Model file for the job. Use its own axes, mm. Coordinates: 2 decimals unless noted, no trailing zeros. Order: outer loops, then holes, each group sorted by start corner. A loop starts at its lowest first (then second) coordinate and runs counter-clockwise, first axis right, second up. Notation, with made-up numbers: M -28,83.5 L 1,83.5 A17 ccw 1,108.5 Z; hole C -9.5,13 d6. An arc over 180 degrees is marked long. Return JSON: item names as keys, results as strings.
Autodesk Inventor part; units mm, degrees
ref_plane "Zplus_face" through (0, 0, 1.5875) normal (0, 0, 1) x (1, 0, 0)
ref_plane "Work Plane_ConnX" through (-32, 0, 0) normal (1, 0, 0) x (0, 1, 0)
ref_plane "Work Plane_ConnY" through (0, 0, 0) normal (0, 1, 0) x (-1, 0, 0)
sketch "AL_spacer_contact_Zminus" plane through (0, 0, 0) normal (0, 0, 1) x (1, 0, 0)
  circle A0 centre (39.5, 39.5) radius 3.175
  circle A1 centre (39.5, -39.5) radius 3.175
  circle A2 centre (-39.5, -39.5) radius 3.175
  circle A3 centre (-39.5, 39.5) radius 3.175
  point P0 (0, 0)
  dimension "d145" = 0
  dimension "d228" = 39.5
  dimension "d229" = 39.5
  dimension "d230" = 39.5
  dimension "d231" = 39.5
  dimension "d232" = 39.5
  dimension "d233" = 39.5
  dimension "d234" = 39.5
  dimension "d235" = 39.5
  dimension "d236" = 6.35
sketch "Delrin_stayout_Zminus" plane through (0, 0, 0) normal (0, 0, 1) x (1, 0, 0)
  line L0 (47.5, 39.5) -> (47.5, 31)
  line L1 (47.5, 31) -> (39.5, 31)
  line L2 (39.5, 31) -> (31, 39.5)
  line L3 (31, 39.5) -> (31, 47.5)
  line L4 (31, 47.5) -> (39.5, 47.5)
  line L5 (39.5, 47.5) -> (47.5, 39.5)
  line L6 (-39.5, 47.5) -> (-47.5, 39.5)
  line L7 (-47.5, 39.5) -> (-47.5, 31)
  line L8 (-47.5, 31) -> (-39.5, 31)
  line L9 (-39.5, 31) -> (-31, 39.5)
  line L10 (-31, 39.5) -> (-31, 47.5)
  line L11 (-31, 47.5) -> (-39.5, 47.5)
  line L12 (47.5, -39.5) -> (39.5, -47.5)
  line L13 (39.5, -47.5) -> (31, -47.5)
  line L14 (31, -47.5) -> (31, -39.5)
  line L15 (31, -39.5) -> (39.5, -31)
  line L16 (39.5, -31) -> (47.5, -31)
  line L17 (47.5, -31) -> (47.5, -39.5)
  line L18 (-39.5, -47.5) -> (-47.5, -39.5)
  line L19 (-47.5, -39.5) -> (-47.5, -31)
  line L20 (-47.5, -31) -> (-39.5, -31)
  line L21 (-39.5, -31) -> (-31, -39.5)
  line L22 (-31, -39.5) -> (-31, -47.5)
  line L23 (-31, -47.5) -> (-39.5, -47.5)
  point P0 (0, 0)
  dimension "d243" = 16.5
  dimension "d244" = 8
  dimension "d245" = 8.5
  dimension "d246" = 16.5
  dimension "d247" = 47.5
  dimension "d248" = 47.5
  dimension "d249" = 47.5
  dimension "d250" = 47.5
  dimension "d251" = 47.5
  dimension "d252" = 47.5
  dimension "d253" = 47.5
  dimension "d254" = 47.5
sketch "Nub_stayout_Zminus" plane through (0, 0, 0) normal (0, 0, 1) x (1, 0, 0)
  line L0 (29, 47.5) -> (39.5, 47.5)
  line L1 (39.5, 47.5) -> (47.5, 39.5)
  line L2 (47.5, 39.5) -> (47.5, 29)
  line L3 (47.5, 29) -> (42, 29)
  line L4 (42, 29) -> (42, 40.4125)
  line L5 (40.4125, 42) -> (29, 42)
  line L6 (29, 42) -> (29, 47.5)
  arc A0 (42, 40.4125) -> (40.4125, 42) centre (40.4125, 40.4125) ccw
  line L7 (-29, 47.5) -> (-39.5, 47.5)
  line L8 (-39.5, 47.5) -> (-47.5, 39.5)
  line L9 (-47.5, 39.5) -> (-47.5, 29)
  line L10 (-47.5, 29) -> (-42, 29)
  line L11 (-42, 29) -> (-42, 40.4125)
  line L12 (-40.4125, 42) -> (-29, 42)
  line L13 (-29, 42) -> (-29, 47.5)
  arc A1 (-40.4125, 42) -> (-42, 40.4125) centre (-40.4125, 40.4125) ccw
  line L14 (-47.5, -29) -> (-42, -29)
  line L15 (-42, -29) -> (-42, -40.4125)
  line L16 (-40.4125, -42) -> (-29, -42)
  line L17 (-29, -42) -> (-29, -47.5)
  line L18 (-29, -47.5) -> (-39.5, -47.5)
  line L19 (-39.5, -47.5) -> (-47.5, -39.5)
  line L20 (-47.5, -39.5) -> (-47.5, -29)
  arc A2 (-42, -40.4125) -> (-40.4125, -42) centre (-40.4125, -40.4125) ccw
  line L21 (47.5, -29) -> (42, -29)
  line L22 (42, -29) -> (42, -40.4125)
  line L23 (40.4125, -42) -> (29, -42)
  line L24 (29, -42) -> (29, -47.5)
  line L25 (29, -47.5) -> (39.5, -47.5)
  line L26 (39.5, -47.5) -> (47.5, -39.5)
  line L27 (47.5, -39.5) -> (47.5, -29)
  arc A3 (40.4125, -42) -> (42, -40.4125) centre (40.4125, -40.4125) ccw
  point P0 (0, 0)
  dimension "d255" = 1.5875
  dimension "d256" = 18.5
  dimension "d257" = 8
  dimension "d258" = 5.5
  dimension "d259" = 47.5
  dimension "d260" = 47.5
  dimension "d264" = 1.5875
  dimension "d265" = 47.5
  dimension "d266" = 47.5
  dimension "d267" = 1.5875
  dimension "d268" = 47.5
  dimension "d269" = 47.5
  dimension "d270" = 1.5875
  dimension "d271" = 47.5
  dimension "d272" = 47.5
ref_plane "Zplus_face" through (0, 0, 1.5875) normal (0, 0, 1) x (1, 0, 0)
sketch "AL_spacer_contact_Zplus" plane through (0, 0, 1.5875) normal (0, 0, 1) x (1, 0, 0)
  circle A0 centre (-39.5, 39.5) radius 3.175
  circle A1 centre (-39.5, -39.5) radius 3.175
  circle A2 centre (39.5, -39.5) radius 3.175
  circle A3 centre (39.5, 39.5) radius 3.175
  point P0 (0, 0)
  dimension "d129" = 39.5
  dimension "d130" = 39.5
  dimension "d131" = 39.5
  dimension "d132" = 39.5
  dimension "d133" = 6.35
sketch "Delrin_stayout_Zplus" plane through (0, 0, 1.5875) normal (0, 0, 1) x (1, 0, 0)
  line L0 (47.5, -31) -> (47.5, -39.5)
  line L1 (47.5, -39.5) -> (39.5, -47.5)
  line L2 (39.5, -47.5) -> (31, -47.5)
  line L3 (31, -47.5) -> (31, -39.5)
  line L4 (31, -39.5) -> (39.5, -31)
  line L5 (39.5, -31) -> (47.5, -31)
  line L6 (47.5, 31) -> (47.5, 39.5)
  line L7 (47.5, 39.5) -> (39.5, 47.5)
  line L8 (39.5, 47.5) -> (31, 47.5)
  line L9 (31, 47.5) -> (31, 39.5)
  line L10 (31, 39.5) -> (39.5, 31)
  line L11 (39.5, 31) -> (47.5, 31)
  line L12 (-39.5, 47.5) -> (-47.5, 39.5)
  line L13 (-47.5, 39.5) -> (-47.5, 31)
  line L14 (-47.5, 31) -> (-39.5, 31)
  line L15 (-39.5, 31) -> (-31, 39.5)
  line L16 (-31, 39.5) -> (-31, 47.5)
  line L17 (-31, 47.5) -> (-39.5, 47.5)
  line L18 (-47.5, -39.5) -> (-39.5, -47.5)
  line L19 (-39.5, -47.5) -> (-31, -47.5)
  line L20 (-31, -47.5) -> (-31, -39.5)
  line L21 (-31, -39.5) -> (-39.5, -31)
  line L22 (-39.5, -31) -> (-47.5, -31)
  line L23 (-47.5, -31) -> (-47.5, -39.5)
  point P0 (0, 0)
  dimension "d115" = 16.5
  dimension "d116" = 16.5
  dimension "d117" = 8
  dimension "d118" = 8.5
  dimension "d121" = 47.5
  dimension "d122" = 47.5
  dimension "d123" = 47.5
  dimension "d124" = 47.5
  dimension "d125" = 47.5
  dimension "d126" = 47.5
  dimension "d127" = 47.5
  dimension "d128" = 47.5
sketch "Nub_stayout_Zplus" plane through (0, 0, 1.5875) normal (0, 0, 1) x (1, 0, 0)
  line L0 (47.5, 29) -> (42, 29)
  line L1 (42, 29) -> (42, 40.4125)
  line L2 (40.4125, 42) -> (29, 42)
  line L3 (29, 42) -> (29, 47.5)
  arc A0 (42, 40.4125) -> (40.4125, 42) centre (40.4125, 40.4125) ccw
  line L4 (29, 47.5) -> (39.5, 47.5)
  line L5 (39.5, 47.5) -> (47.5, 39.5)
  line L6 (47.5, 39.5) -> (47.5, 29)
  line L7 (-39.5, 47.5) -> (-29, 47.5)
  line L8 (-29, 47.5) -> (-29, 42)
  line L9 (-29, 42) -> (-40.4125, 42)
  line L10 (-42, 40.4125) -> (-42, 29)
  line L11 (-42, 29) -> (-47.5, 29)
  line L12 (-47.5, 29) -> (-47.5, 39.5)
  line L13 (-47.5, 39.5) -> (-39.5, 47.5)
  arc A1 (-40.4125, 42) -> (-42, 40.4125) centre (-40.4125, 40.4125) ccw
  line L14 (-47.5, -29) -> (-47.5, -39.5)
  line L15 (-47.5, -39.5) -> (-39.5, -47.5)
  line L16 (-39.5, -47.5) -> (-29, -47.5)
  line L17 (-29, -47.5) -> (-29, -42)
  line L18 (-29, -42) -> (-40.4125, -42)
  line L19 (-42, -40.4125) -> (-42, -29)
  line L20 (-42, -29) -> (-47.5, -29)
  arc A2 (-42, -40.4125) -> (-40.4125, -42) centre (-40.4125, -40.4125) ccw
  line L21 (29, -47.5) -> (39.5, -47.5)
  line L22 (39.5, -47.5) -> (47.5, -39.5)
  line L23 (47.5, -39.5) -> (47.5, -29)
  line L24 (47.5, -29) -> (42, -29)
  line L25 (42, -29) -> (42, -40.4125)
  line L26 (40.4125, -42) -> (29, -42)
  line L27 (29, -42) -> (29, -47.5)
  arc A3 (40.4125, -42) -> (42, -40.4125) centre (40.4125, -40.4125) ccw
  point P0 (0, 0)
  dimension "d146" = 1.5875
  dimension "d147" = 5.5
  dimension "d149" = 18.5
  dimension "d150" = 8
  dimension "d151" = 47.5
  dimension "d152" = 47.5
  dimension "d153" = 1.5875
  dimension "d154" = 47.5
  dimension "d155" = 47.5
  dimension "d156" = 1.5875
  dimension "d157" = 47.5
  dimension "d158" = 47.5
  dimension "d159" = 1.5875
  dimension "d160" = 47.5
  dimension "d161" = 47.5
sketch "Sketch1" plane through (0, 0, 0) normal (0, 0, 1) x (1, 0, 0)
  line L0 (-47.5, 47.5) -> (47.5, 47.5)
  line L1 (47.5, 47.5) -> (47.5, -47.5)
  line L2 (47.5, -47.5) -> (-47.5, -47.5)
  line L3 (-47.5, -47.5) -> (-47.5, 47.5)
  point P0 (0, 0)
  dimension "d0" = 95
  dimension "d1" = 95
  dimension "d2" = 47.5
  dimension "d3" = 47.5
extrude "Extrusion1" add sketch "Sketch1" along normal blind 1.5875
chamfer "Chamfer2" distance 11 angle 45 4 edges at (-47.5, -47.5, 0.7937) (47.5, -47.5, 0.7937) (47.5, 47.5, 0.7937) (-47.5, 47.5, 0.7937)
ref_plane "Work Plane_ConnX" through (-32, 0, 0) normal (1, 0, 0) x (0, 1, 0)
ref_plane "Work Plane_ConnY" through (0, 0, 0) normal (0, 1, 0) x (-1, 0, 0)
sketch "Sketch9" plane through (0, 0, 1.5875) normal (0, 0, 1) x (1, 0, 0)
  line L0 (47.5, 47.5) -> (47.5, -47.5)
  line L1 (58.5598, -32) -> (-58.5598, -32)
  circle A0 centre (-2.667, -21.9289) radius 0.4445
  circle A1 centre (-2.667, -42.0711) radius 0.4445
  line L2 (0, 26.5598) -> (0, -90.5598) construction
  point P0 (0, 0)
  point P1 (0, -32)
  dimension "d134" = 20.1422
  dimension "d136" = 2.667
  dimension "d138" = 0.889
  dimension "d141" = 180
  dimension "d350" = 32
  dimension "d351" = 0
extrude "Holes_Conn_Zminus" cut sketch "Sketch9" against normal through all
sketch "Sketch22" plane through (0, 0, 1.5875) normal (0, 0, 1) x (1, 0, 0)
  line L0 (47.5, 36.5) -> (47.5, -36.5)
  line L1 (0, -1.0026) -> (0, -62.9974) construction
  line L2 (62.8115, -32) -> (-62.8115, -32)
  circle A0 centre (2.032, -22.7545) radius 0.4445
  circle A1 centre (2.032, -41.2455) radius 0.4445
  point P0 (0, 0)
  point P1 (0, -32)
  dimension "d282" = 180
  dimension "d283" = 18.491
  dimension "d284" = 0.889
  dimension "d285" = 2.032
  dimension "d352" = 32
  dimension "d353" = 0
extrude "Holes_Conn_Zplus" cut sketch "Sketch22" against normal through all
hole "Hole5" at (39.5, 39.5, 1.5875) direction (0, 0, -1) diameter 3.2 end through all
mirror "Mirror5" about plane through (0, 0, 0) normal (1, 0, 0) of "Hole5"
mirror "Mirror6" about plane through (0, 0, 0) normal (0, 1, 0) of "Hole5", "Mirror5"
sketch "Sketch25" plane through (0, 0, 1.5875) normal (0, 0, 1) x (1, 0, 0)
  circle A0 centre (-39.5, -39.5) radius 1.6
  circle A1 centre (39.5, -39.5) radius 1.6
  circle A2 centre (-39.5, 39.5) radius 1.6
  circle A3 centre (39.5, 39.5) radius 1.6
  line L0 (36.5, -47.5) -> (-36.5, -47.5)
  line L1 (0, 0) -> (0, -59.2198)
  line L2 (8, -47.5) -> (8, -15.5)
  line L3 (8, -15.5) -> (-8, -15.5)
  line L4 (-8, -15.5) -> (-8, -47.5)
  line L5 (-8, -47.5) -> (-62.7516, -61.7336)
  line L6 (-62.7516, -61.7336) -> (-64.2933, 68.2222)
  line L7 (-64.2933, 68.2222) -> (58.3572, 62.5728)
  line L8 (58.3572, 62.5728) -> (56.5848, -69.017)
  line L9 (56.5848, -69.017) -> (8, -47.5)
  dimension "d362" = 16
  dimension "d363" = 32
extrude "Extrusion9" [suppressed]
sketch "Sketch26" plane through (0, 0, 1.5875) normal (0, 0, 1) x (1, 0, 0)
  line L0 (-47.5, -36.5) -> (-47.5, 36.5)
  line L1 (36.5, -47.5) -> (-36.5, -47.5)
  line L2 (47.5, 36.5) -> (47.5, -36.5)
  line L3 (-36.5, 47.5) -> (36.5, 47.5)
  line L4 (47.5, 47.5) -> (47.5, -47.5) construction
  line L5 (47.5, -47.5) -> (-47.5, -47.5) construction
  line L6 (-47.5, -47.5) -> (-47.5, 47.5) construction
  line L7 (-47.5, 47.5) -> (47.5, 47.5) construction
  point P0 (0, 0)
decal "Decal1"
sketch "Sketch27" plane through (0, 0, 0) normal (0, 0, -1) x (-1, 0, 0)
  line L0 (36.5, 47.5) -> (-36.5, 47.5)
  line L1 (-47.5, 36.5) -> (-47.5, -36.5)
  line L2 (-36.5, -47.5) -> (36.5, -47.5)
  line L3 (47.5, -36.5) -> (47.5, 36.5)
  line L4 (47.5, 47.5) -> (47.5, -47.5) construction
  line L5 (47.5, -47.5) -> (-47.5, -47.5) construction
  line L6 (-47.5, -47.5) -> (-47.5, 47.5) construction
  line L7 (-47.5, 47.5) -> (47.5, 47.5) construction
  point P0 (0, 0)
decal "Decal2"
hole "Hole13" at (-9.5016, 34.4901, 1.5875) direction (0, 0, -1) diameter 1.999 end through all
hole "Hole14" at (9.4976, 34.4901, 1.5875) direction (0, 0, -1) diameter 1.999 end through all
hole "Hole15" at (-5.2598, 38.9935, 1.5875) direction (0, 0, -1) diameter 3.175 end through all
properties part number "PCB_Batt1" material "FR4"
Item 1: Saw through at D-D (z = 1.2). Count the separate pieces of the cut face and the enclosed holes in it, and give its area (3 significant figures).
Check result:
{"separate pieces": "1", "enclosed holes": "11", "area": "8,730 mm2"}
Item 2: Pull direction Y, two halves, no side cores. Call faces 1 (the cylindrical face through (-38.08, 38.76, 0.78)), 2 (the flat face through (-42, -42, 1)), 3 (the flat face through (-42, 42, 1)): +Y half, -Y half, draft (parallel to the pull), parting line (faces both ways), or undercut.
Check result:
{"face 1": "undercut", "face 2": "-Y half", "face 3": "+Y half"}
Item 3: Saw through at A-A (y = -39.5). Write the cut outline in (x, z).
Check result:
{"outline": "M -44.5,0 L -41.1,0 L -41.1,1.59 L -44.5,1.59 Z; M -37.9,0 L 37.9,0 L 37.9,1.59 L -37.9,1.59 Z; M 41.1,0 L 44.5,0 L 44.5,1.59 L 41.1,1.59 Z"}
Item 4: Wall check: line 1 (X direction, y = -39.5, z = 1.2); line 2 (Y direction, x = -9.5, z = 1); line 3 (X direction, y = 39.5, z = 0.95). Give the ranges that are in metal, low to high.
Check result:
{"line 1": "x = -44.5 to -41.1, -37.9 to 37.9, 41.1 to 44.5", "line 2": "y = -47.5 to 33.49, 35.49 to 47.5", "line 3": "x = -44.5 to -41.1, -37.9 to -6.76, -3.76 to 37.9, 41.1 to 44.5"}
Item 5: Saw through at C-C (y = 39.5). Write the cut outline in (x, z), and give its area (3 significant figures).
Check result:
{"outline": "M -44.5,0 L -41.1,0 L -41.1,1.59 L -44.5,1.59 Z; M -37.9,0 L -6.76,0 L -6.76,1.59 L -37.9,1.59 Z; M -3.76,0 L 37.9,0 L 37.9,1.59 L -3.76,1.59 Z; M 41.1,0 L 44.5,0 L 44.5,1.59 L 41.1,1.59 Z", "area": "126 mm2"}
